from build123d import *

# Parameters (mm, degrees)
ESQUISSE1_R             = 75
ESQUISSE1_R_2           = 55
BOSS_EXTRU_3_DEPTH      = 18
ESQUISSE6_R             = 60
ESQUISSE6_R_2           = 55
ENL_V_MAT_EXTRU_2_DEPTH = 4
ESQUISSE5_R             = 3.175
ENL_V_MAT_EXTRU_1_DEPTH = 3.15
ESQUISSE9_R             = 3.175
ENL_V_MAT_EXTRU_3_DEPTH = 3.15


with BuildPart() as part:
    # Esquisse1 → Boss.-Extru.3 (new body)
    with BuildSketch(Plane(origin=(0, 0, 0), x_dir=(1, 0, 0), z_dir=(0, 1, 0))):
        with Locations(Location((0, 0, 0), (0, 0, 270))):  # turned: the seam where the file's is
            Circle(ESQUISSE1_R)
        with Locations(Location((0, 0, 0), (0, 0, 270))):  # turned: the seam where the file's is
            Circle(ESQUISSE1_R_2, mode=Mode.SUBTRACT)
    extrude(amount=BOSS_EXTRU_3_DEPTH)

    # Esquisse6 → Enlèv. mat.-Extru.2 (cut)
    with BuildSketch(Plane(origin=(0, 18, 0), x_dir=(1, 0, 0), z_dir=(0, 1, 0))):
        with Locations(Location((0, 0, 0), (0, 0, 270))):  # turned: the seam where the file's is
            Circle(ESQUISSE6_R)
        with Locations(Location((0, 0, 0), (0, 0, 270))):  # turned: the seam where the file's is
            Circle(ESQUISSE6_R_2, mode=Mode.SUBTRACT)
    extrude(amount=-ENL_V_MAT_EXTRU_2_DEPTH, mode=Mode.SUBTRACT)

    # Esquisse5 → Enlèv. mat.-Extru.1 (cut)
    with BuildSketch(Plane(origin=(0, 18, 0), x_dir=(1, 0, 0), z_dir=(0, 1, 0))):
        with Locations(Location((-59.441823855, 26.299611723, 0), (0, 0, 270))):  # turned: the seam where the file's is
            Circle(ESQUISSE5_R)
        with Locations(Location((52.497043789, 38.328323645, 0), (0, 0, 270))):  # turned: the seam where the file's is
            Circle(ESQUISSE5_R)
        with Locations(Location((6.944780066, -64.627935367, 0), (0, 0, 270))):  # turned: the seam where the file's is
            Circle(ESQUISSE5_R)
    extrude(amount=-ENL_V_MAT_EXTRU_1_DEPTH, mode=Mode.SUBTRACT)

    # Esquisse9 → Enlèv. mat.-Extru.3 (cut)
    with BuildSketch(Plane.XZ):
        with Locations(Location((59.441823855, 26.299611723, 0), (0, 0, 270))):  # turned: the seam where the file's is
            Circle(ESQUISSE9_R)
        with Locations(Location((-6.944780066, -64.627935367, 0), (0, 0, 270))):  # turned: the seam where the file's is
            Circle(ESQUISSE9_R)
        with Locations(Location((-52.497043789, 38.328323645, 0), (0, 0, 270))):  # turned: the seam where the file's is
            Circle(ESQUISSE9_R)
    extrude(amount=-ENL_V_MAT_EXTRU_3_DEPTH, mode=Mode.SUBTRACT)


solid = part.part
The model under review builds one solid part; all positions refer to its coordinate system, in mm. A direction names the side the tool comes from. Give positions to 0.01 mm unless a question says otherwise; leave off trailing zeros. Loops run counter-clockwise (first coordinate to the right, second up) from the corner with the lowest first, then second, coordinate; pieces in that order, holes last. Notation, with made-up numbers: (58, 31.25) -> (113, 31.25) arc R17 ccw to (113, 44.25) -> close; hole circle Ø7 at (-13.75, 5). An arc over 180 degrees is marked (long way). Put each result on its own line as item: value. Start each with the question number.
1. We need section B-B on z = 0. State the section outline as (x, y) points.
2. For faces 1 (the face through (-48.794, 6.902, 25.379)), 2 (the face through (53, 14.85, -38)), 3 (the face through (57.51, 1.55, 28.82)), list the 3-axis set-ups (+Z, -Z, +X, -X, +Y, -Y) from which the entire face can be reached by the end or side of a thin tool; tool diameter is ignored.
3. Mouldability with a two-part tool opening along Y and no side actions: class faces 4 (the face through (-7, 3.15, -65)), 5 (the face through (-54.429, 1.553, 40.848)), 6 (the face through (50, 18, -34)) as released by +Y, released by -Y, zero draft, split by the parting line, or undercut.
4. Clearance check with flat-ended pins moving along their axes: P1, Ø5, axis at y = 10, z = -52, coming from the +X side; P2, Ø4, axis at x = -59.44, z = -26.3, coming from the +Y side; P3, Ø8, axis at y = 10, z = 8.5, coming from the +X side. State where each tip first meets the part, or that it passes through.
5. We need section C-C on y = 11.25. State the section outline as (x, z) points, then the cut area to 3 significant figures.
6. Wall thickness on probe 1 along X at (y, z) = (15.2, 0); probe 2 along Z at (x, y) = (50.5, 15.75); probe 3 along X at (y, z) = (5.25, 0): over which ranges is each line inside the solid? List them lowest first.
7. We need section A-A on x = 0. State the section outline as (y, z) points, then the cut area to 3 significant figures.
Determined:
1. outline: (-75, 0) -> (-55, 0) -> (-55, 14) -> (-60, 14) -> (-60, 18) -> (-75, 18) -> close; (55, 0) -> (75, 0) -> (75, 18) -> (60, 18) -> (60, 14) -> (55, 14) -> close
2. face 1: +Y, -Y
2. face 2: +Y
2. face 3: -Y
3. face 4: released by -Y
3. face 5: zero draft
3. face 6: released by +Y
4. P1: x = 56.34
4. P2: y = 14.85
4. P3: x = 74.86
5. outline: circle Ø150 at (0, 0); hole circle Ø110 at (0, 0)
5. area: 8,170 mm^2
6. probe 1: -75 to -60, 60 to 75
6. probe 2: -55.45 to -40.8, -35.86 to -32.4, 32.4 to 55.45
6. probe 3: -75 to -55, 55 to 75
7. outline: (0, -75) -> (18, -75) -> (18, -60) -> (14, -60) -> (14, -55) -> (0, -55) -> close; (0, 55) -> (14, 55) -> (14, 60) -> (18, 60) -> (18, 75) -> (0, 75) -> close
7. area: 680 mm^2
